Source: three-view drawing plus pictorial views. Frame: mm from the lowest corner of the part. Give positions to 0.01 mm unless a question says otherwise; leave off trailing zeros. Order: outer loops, then holes, each group sorted by start corner. A loop starts at its lowest first (then second) coordinate and runs counter-clockwise, first axis right, second up.
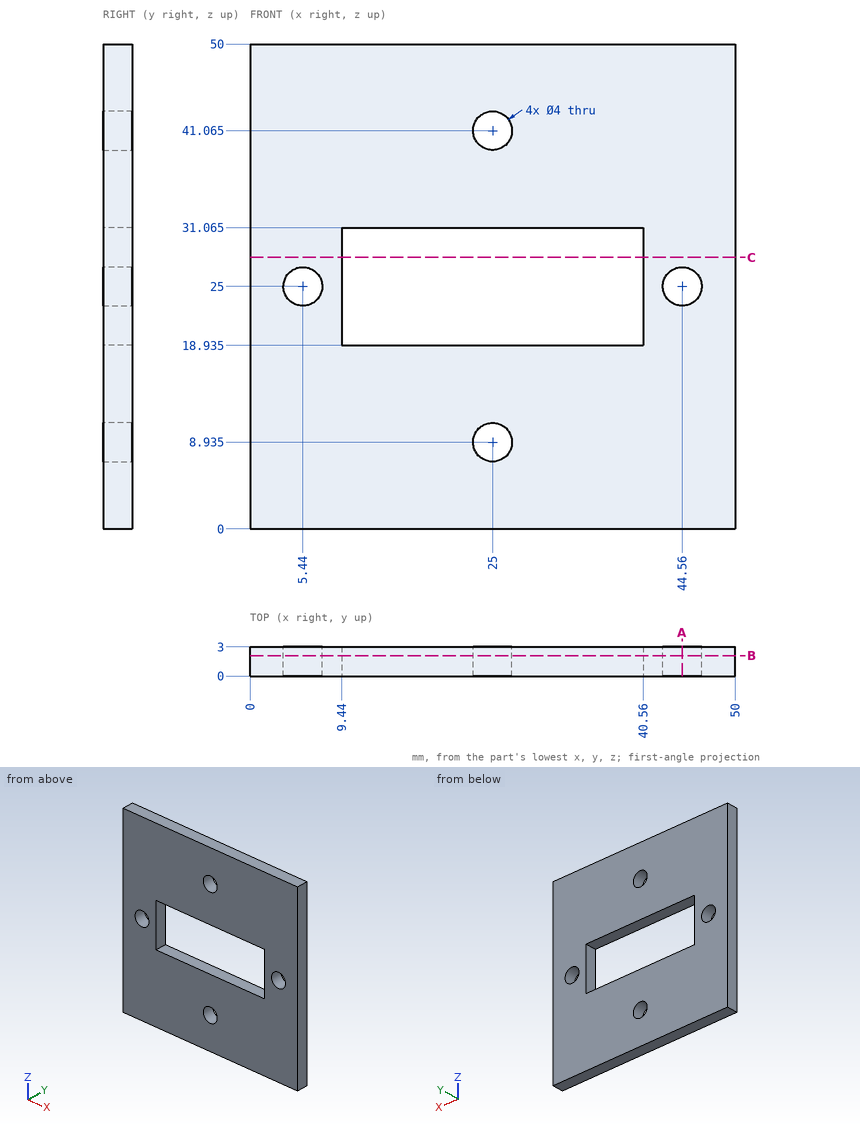
(1) Section B-B, the plane y = 2.1. Return loops of the section in (x, z) (3 decimals).
(2) Section A-A, the plane x = 44.56. Return loops of the section in (y, z), plus the area to 3 significant figures.
(3) Section C-C, the plane z = 28. Return loops of the section in (x, y).
(4) Line query: line 1 along X through (y, z) = (2.25, 25); line 2 along X through (y, z) = (1.75, 9); line 3 along Z through (x, y) = (37.5, 0.9) (3 decimals). Output: solid intervals per line, ascending.
Checks:
1. outline: (0, 0) - (50, 0) - (50, 50) - (0, 50) - close; hole circle Ø4 at (5.44, 25); hole (9.44, 18.935) - (40.56, 18.935) - (40.56, 31.065) - (9.44, 31.065) - close; hole circle Ø4 at (25, 8.935); hole circle Ø4 at (25, 41.065); hole circle Ø4 at (44.56, 25)
2. outline: (0, 0) - (3, 0) - (3, 23) - (0, 23) - close; (0, 27) - (3, 27) - (3, 50) - (0, 50) - close
2. area: 138 mm2
3. outline: (0, 0) - (9.44, 0) - (9.44, 3) - (0, 3) - close; (40.56, 0) - (50, 0) - (50, 3) - (40.56, 3) - close
4. line 1: x = 0 to 3.44, 7.44 to 9.44, 40.56 to 42.56, 46.56 to 50
4. line 2: x = 0 to 23, 27 to 50
4. line 3: z = 0 to 18.935, 31.065 to 50
